Here's how the part is built. I have some questions about the finished solid (model axes, mm). Give positions to 0.01 mm unless a question says otherwise; leave off trailing zeros. Order: outer loops, then holes, each group sorted by start corner. A loop starts at its lowest first (then second) coordinate and runs counter-clockwise, first axis right, second up. Notation, with made-up numbers: M 36,2 L 75,2 A20 cw 75,13 Z; hole C 41,14 d10. An arc over 180 degrees is marked long. Use CSV: the item, a comma, the result in double quotes. Start each with the question number.
```python
from build123d import *

# Parameters (mm, degrees)
F0_R     = 35
F1_DEPTH = 20
F2_R     = 27.5
F3_DEPTH = 25
F4_R     = 2
F5_R     = 2


with BuildPart() as f1:
    # F0 (on Top) → F1 (new body)
    with BuildSketch(Plane.XY):
        Circle(F0_R)
    extrude(amount=F1_DEPTH)

    # F2 (on face) → F3 (cut)
    with BuildSketch(Plane.XY.offset(20)):
        Circle(F2_R)
    extrude(amount=-F3_DEPTH, mode=Mode.SUBTRACT)

    # F4
    f4_edges = [f1.edges().sort_by_distance(p)[0] for p in [
        (-27.5, 0, 20),
        (-27.5, 0, 0),
    ]]
    fillet(f4_edges, radius=F4_R)

    # F5
    f5_edges = [f1.edges().sort_by_distance(p)[0] for p in [
        (-35, 0, 20),
        (-35, 0, 0),
    ]]
    fillet(f5_edges, radius=F5_R)


solid = f1.part
```
Q1. Imagine slicing it at C-C, the plane z = 11.25. Please give me the cut outline in (x, y).
Q2. I need wall thicknesses on line 1 (Y direction, x = 0, z = 8); line 2 (Y direction, x = 2, z = 8.25); line 3 (X direction, y = -18.5, z = 2). Which ranges of each line are inside material? Lowest first, please. Write a range as [from, to].
Q3. We'd pull the mould along Y, two halves only. Please class faces 1 (the face through (-5.961, -26.846, 10.112)), 2 (the face through (-25, -17, 20)), 3 (the face through (-28, -21, 10)): pulls with the +Y half, pulls with the -Y half, needs draft (parallel to the pull), parting line crosses it, or undercut.
Q4. For P1, Ø8, axis at x = 19, z = 17.5, coming from the +Y side; P2, Ø6, axis at x = 25, z = 12, coming from the +Y side; P3, Ø12, axis at x = 9, z = 7, coming from the +Y side, each with a flat end and sliding along its axis, tell me the tip position at first contact or that it passes through.
Q5. Imagine slicing it at A-A, the plane y = 0. Please give me the cut outline in (x, z), then the cut area to 3 significant figures.
Reply:
1,outline,"C 0,0 d70; hole C 0,0 d55"
2,line 1,"y = [-35, -27.5], [27.5, 35]"
2,line 2,"y = [-34.94, -27.43], [27.43, 34.94]"
2,line 3,"x = [-29.71, -20.35], [20.35, 29.71]"
3,face 1,"undercut"
3,face 2,"needs draft"
3,face 3,"parting line crosses it"
4,P1,"stops at y = 31.62"
4,P2,"stops at y = 27.22"
4,P3,"stops at y = 34.87"
5,outline,"M -35,2 A2 ccw -33,0 L -29.5,0 A2 ccw -27.5,2 L -27.5,18 A2 ccw -29.5,20 L -33,20 A2 ccw -35,18 Z; M 27.5,2 A2 ccw 29.5,0 L 33,0 A2 ccw 35,2 L 35,18 A2 ccw 33,20 L 29.5,20 A2 ccw 27.5,18 Z"
5,area,"293 mm^2"
